The model under review builds one solid part; all positions refer to its coordinate system, in mm. A direction names the side the tool comes from. Coordinates: 2 decimals unless noted, no trailing zeros. Order: outer loops, then holes, each group sorted by start corner. A loop starts at its lowest first (then second) coordinate and runs counter-clockwise, first axis right, second up. Notation, with made-up numbers: (54, -32.75) - (94, -32.75) arc R16 cw to (94, -20.75) - close; hole circle Ø1 at (4.25, 60.5). An arc over 180 degrees is marked (long way). Answer in a Markdown table with one row per item.
```python
from build123d import *

# Parameters (mm, degrees)
SKETCH1_W                  = 101.6
SKETCH1_H                  = 38.1
SKETCH1_R                  = 2.5796875
BOSS_EXTRUDE1_DEPTH        = 1.5875
SKETCHED_START             = -19.05
SKETCHED_BEND1_DEPTH       = 38.1
SKETCHED_BEND1_2_DEPTH     = 16.4703124
SKETCHED_START_2           = 2.5796876
SKETCHED_BEND1_3_DEPTH     = 16.4703124
SKETCHED_START_3           = -2.5796876
SKETCHED_BEND1_4_DEPTH     = 5.1593752
SKETCHED_START_4           = 3.905760394
SKETCHED_BEND1_5_OUTLINE_R = 2.5796875
SKETCHED_BEND1_5_DEPTH     = 1.5875


with BuildPart() as part:
    # Sketch1 → Boss-Extrude1 (new body)
    with BuildSketch(Plane(origin=(0, 0, 0), x_dir=(1, 0, 0), z_dir=(0, 1, 0))):
        Rectangle(SKETCH1_W, SKETCH1_H)
        with Locations(Location((-38.1, 0, 0), (0, 0, 270))):
            Circle(SKETCH1_R, mode=Mode.SUBTRACT)
        with Locations(Location((38.1, 0, 0), (0, 0, 270))):
            Circle(SKETCH1_R, mode=Mode.SUBTRACT)
    extrude(amount=BOSS_EXTRUDE1_DEPTH)

    # Sketched Bend1: read off the stored shape, not the designer's step
    # Sketched Bend1 outline → Sketched Bend1 (cut)
    with BuildSketch(Plane.XY.offset(SKETCHED_START)):
        with BuildLine():
            Line((50.8, 1.5875), (-4.318797944, 1.5875))
            ThreePointArc((-4.318797944, 1.5875), (-7.140118794, 0.403914791), (-10.172869711, 0))
            Line((-10.172869711, 0), (50.8, 0))
            Line((50.8, 0), (50.8, 1.5875))
        make_face()
    extrude(amount=SKETCHED_BEND1_DEPTH, mode=Mode.SUBTRACT)

    # Sketched Bend1 2 outline → Sketched Bend1 2 (add)
    with BuildSketch(Plane.XY.offset(SKETCHED_START)):
        with BuildLine():
            Line((-13.21677824, 53.316366943), (-0.662304548, 14.677669944))
            ThreePointArc((-0.662304548, 14.677669944), (-2.082699768, 5.709647478), (-10.172869711, 1.5875))
            Line((-10.172869711, 1.5875), (-4.318797944, 1.5875))
            ThreePointArc((-4.318797944, 1.5875), (0.657447044, 7.467500578), (0.847497671, 15.168234422))
            Line((0.847497671, 15.168234422), (-11.706976021, 53.806931422))
            Line((-11.706976021, 53.806931422), (-13.21677824, 53.316366943))
        make_face()
    extrude(amount=SKETCHED_BEND1_2_DEPTH)

    # Sketched Bend1 3 outline → Sketched Bend1 3 (add)
    with BuildSketch(Plane.XY.offset(SKETCHED_START_2)):
        with BuildLine():
            Line((-13.21677824, 53.316366943), (-0.662304548, 14.677669944))
            ThreePointArc((-0.662304548, 14.677669944), (-2.082699768, 5.709647478), (-10.172869711, 1.5875))
            Line((-10.172869711, 1.5875), (-4.318797944, 1.5875))
            ThreePointArc((-4.318797944, 1.5875), (0.657447044, 7.467500578), (0.847497671, 15.168234422))
            Line((0.847497671, 15.168234422), (-11.706976021, 53.806931422))
            Line((-11.706976021, 53.806931422), (-13.21677824, 53.316366943))
        make_face()
    extrude(amount=SKETCHED_BEND1_3_DEPTH)

    # Sketched Bend1 4 outline → Sketched Bend1 4 (add)
    with BuildSketch(Plane.XY.offset(SKETCHED_START_3)):
        with BuildLine():
            Line((-13.21677824, 53.316366943), (-0.662304548, 14.677669944))
            ThreePointArc((-0.662304548, 14.677669944), (-2.082699768, 5.709647478), (-10.172869711, 1.5875))
            Line((-10.172869711, 1.5875), (-4.318797944, 1.5875))
            ThreePointArc((-4.318797944, 1.5875), (0.657447044, 7.467500578), (0.847497671, 15.168234422))
            Line((0.847497671, 15.168234422), (-11.706976021, 53.806931422))
            Line((-11.706976021, 53.806931422), (-13.21677824, 53.316366943))
        make_face()
    extrude(amount=SKETCHED_BEND1_4_DEPTH)

    # Sketched Bend1 5 outline → Sketched Bend1 5 (cut)
    with BuildSketch(Plane(origin=(0, 0, 0), x_dir=(-0.30901699437495117, 0.9510565162951524, 0), z_dir=(0.9510565162951524, 0.3090169943749511, 0)).offset(SKETCHED_START_4)):
        with Locations((42.091087294, 0)):
            Circle(SKETCHED_BEND1_5_OUTLINE_R)
    extrude(amount=SKETCHED_BEND1_5_DEPTH, mode=Mode.SUBTRACT)


solid = part.part
```
Item 1: Clearance check with flat-ended pins moving along their axes: pin 1 Ø1 at (x, z) = (-16, -7.5) entering from +Y; pin 2 Ø1.5 at (y, z) = (32, -11) entering from +X; pin 3 Ø1.5 at (y, z) = (22.5, 1) entering from +X; pin 4 Ø4 at (x, z) = (-38.1, 0) entering from -Y. State where each tip first meets the part, or that it passes through.
Check values:
| item | result |
|---|---|
| pin 1 | y = 1.59 |
| pin 2 | x = -4.38 |
| pin 3 | x = -1.29 |
| pin 4 | through |
Item 2: We need section B-B, the plane z = 9.5. Write out the cut boundary in (x, y) (1 decimal), then the cut area to 3 significant figures.
Check values:
| item | result |
|---|---|
| outline | (-50.8, 0) - (-10.2, 0) arc R11.6 ccw to (0.8, 15.2) - (-11.7, 53.8) - (-13.2, 53.3) - (-0.7, 14.7) arc R10 cw to (-10.2, 1.6) - (-50.8, 1.6) - close |
| area | 161 mm^2 |
Item 3: We need section C-C, the plane z = 0. Write out the cut boundary in (x, y) (1 decimal), then the cut area to 3 significant figures.
Check values:
| item | result |
|---|---|
| outline | (-50.8, 0) - (-40.7, 0) - (-40.7, 1.6) - (-50.8, 1.6) - close; (-35.5, 0) - (-10.2, 0) arc R11.6 ccw to (0.8, 15.2) - (-7, 39.3) - (-8.5, 38.8) - (-0.7, 14.7) arc R10 cw to (-10.2, 1.6) - (-35.5, 1.6) - close; (-13.2, 53.3) - (-10.1, 43.7) - (-8.6, 44.2) - (-11.7, 53.8) - close |
| area | 145 mm^2 |
Item 4: Tool access review of faces 4 (the face through (-7.03, 34.27, -0.27)), 5 (the face through (-17, 1, -19.05)): name each direction out of +Z, -Z, +X, -X, +Y, -Y from which nothing blocks a thin tool from reaching the whole face with its end or side.
Check values:
| item | result |
|---|---|
| face 4 | +Z, -Z, -X |
| face 5 | -Z, +X, -X, +Y, -Y |
Item 5: Mouldability with a two-part tool opening along X and no side actions: class faces 1 (the face through (-31, 0, 0)), 2 (the face through (-9.284, 43.746, -0.988)), 3 (the face through (-40.62, 0.78, -0.56)) as +X half, -X half, draft (parallel to the pull), parting line (faces both ways), or undercut.
Check values:
| item | result |
|---|---|
| face 1 | draft |
| face 2 | parting line |
| face 3 | undercut |
Item 6: We need section D-D, the plane x = -15. Write out the cut boundary in (y, z).
Check values:
| item | result |
|---|---|
| outline | (0, -19.05) - (1.59, -19.05) - (1.59, 19.05) - (0, 19.05) - close |
Item 7: We need section A-A, the plane x = -38.1. Write out the cut boundary in (y, z).
Check values:
| item | result |
|---|---|
| outline | (0, -19.05) - (1.59, -19.05) - (1.59, -2.58) - (0, -2.58) - close; (0, 2.58) - (1.59, 2.58) - (1.59, 19.05) - (0, 19.05) - close |
Item 8: To check wall thickness, follow line 1 (Z direction, x = -38, y = 1); line 2 (Y direction, x = -48.5, z = 14.5); line 3 (X direction, y = 0.9, z = 0). State the ranges of each line that lie inside material, in increasing order. Write a range as from..to.
Check values:
| item | result |
|---|---|
| line 1 | -19.05..-2.58, 2.58..19.05 |
| line 2 | 0..1.59 |
| line 3 | -50.8..-40.68, -35.52..-5.7 |
